from build123d import *

# Parameters (mm, degrees)
F0_R     = 25.4
F1_DEPTH = 6.35
F3_DEPTH = 12.7
F5_COUNT = 6
F6_R     = 5.616515
F7_DEPTH = 12.7


with BuildPart() as f1:
    # F0 (on Top) → F1 (new body, symmetric)
    with BuildSketch(Plane.XY):
        Circle(F0_R)
    extrude(amount=F1_DEPTH, both=True)

    # F2 (on face) → F3 (join)
    with BuildSketch(Plane(origin=(0, 0, -6.35), x_dir=(1, 0, 0), z_dir=(0, 0, -1))):
        with BuildLine():
            Line((-6.574004, 24.534516), (0, 24.477616))
            Line((0, 24.477616), (0, 25.4))
            ThreePointArc((0, 25.4), (-3.315365, 25.182699), (-6.574004, 24.534516))
        make_face()
        with BuildLine():
            Line((0, 25.4), (0, 24.477616))
            Line((0, 24.477616), (6.543582, 24.420979))
            Line((6.543582, 24.420979), (6.574004, 24.534516))
            ThreePointArc((6.574004, 24.534516), (3.315365, 25.182699), (0, 25.4))
        make_face()
        with BuildLine():
            Line((-6.486069, 34.694135), (-6.574004, 24.534516))
            ThreePointArc((-6.574004, 24.534516), (-3.315365, 25.182699), (0, 25.4))
            ThreePointArc((0, 25.4), (3.315365, 25.182699), (6.574004, 24.534516))
            Line((6.574004, 24.534516), (7.085632, 34.576668))
            Line((7.085632, 34.576668), (-6.486069, 34.694135))
        make_face()
    extrude(amount=-F3_DEPTH)

    # F5: F1 ×6 about axis
    f5_axis = Axis((0, 0, 22.241494), (0, 0, 1))


with BuildPart() as f1_1:
    add(f1.part)
    for i in range(1, F5_COUNT):
        add(f1.part.rotate(f5_axis, i * 360 / F5_COUNT))

    # F6 (on face) → F7 (cut)
    with BuildSketch(Plane.XY.offset(6.35)):
        with Locations((-0.299782, 0)):
            Circle(F6_R)
    extrude(amount=-F7_DEPTH, mode=Mode.SUBTRACT)


solid = f1_1.part
Input: part model. Units: mm. Frame: model coordinates. A direction names the side the tool comes from. Round coordinates to 2 decimals unless told otherwise and drop trailing zeros. Order: outer loops, then holes, each group sorted by start corner. A loop starts at its lowest first (then second) coordinate and runs counter-clockwise, first axis right, second up. Notation, with made-up numbers: (-12.75, -20.5) - (-1.75, -20.5) arc R11 cw to (-1.75, -4.5) - close; hole circle Ø5 at (67.5, -28). An arc over 180 degrees is marked (long way). Answer as a JSON object with one key per item and string values. Group by question number.
(1) Pin query (flat end, axial travel): P1, Ø6.5, axis at x = -0.3, y = 0, coming from the -Z side; P2, Ø1.5, axis at x = -19.5, z = 5, coming from the +Y side; P3, Ø5, axis at y = 4, z = 4.5, coming from the -X side; P4, Ø4, axis at y = -16.5, z = 5, coming from the -X side. Return the tip coordinate at first contact, or that it passes through.
(2) Cut plane A-A (y = 0). Return loops of the section in (x, z), then the cut area to 4 significant figures.
(3) Material intervals for probe 1 along X at (y, z) = (-22, 5.75); probe 2 along Y at (x, z) = (2, 2.25); probe 3 along Y at (x, z) = (28, 4.75) (3 decimals), sorted ascending. Write a range as from..to.
(4) Cut plane C-C (x = 4). Return loops of the section in (y, z), then the cut area to 3 significant figures.
(5) Draft query along Y for faces 6 (the face through (-1.03, 5.57, 0.09)), 7 (the face through (30.19, -16.98, -0.09)), 8 (the face through (22.122, 20.654, -0.089)). Return one class per face: released by +Y, released by -Y, zero draft, split by the parting line, or undercut.
(6) Cut plane D-D (x = 20). Return loops of the section in (y, z).
(7) Reachability of faces 1 (the face through (-28.95, 8.83, -0.09)), 2 (the face through (28.95, -8.83, -0.09)), 3 (the face through (29.797, 17.659, -0.089)), 4 (the face through (12.78, 21.95, 0.09)), 5 (the face through (-12.78, -21.95, 0.09)) from +Z, -Z, +X, -X, +Y, -Y: full face, straight path, thin tool, end or side. Return the list, or none.
(8) Cut plane B-B (z = 0). Return loops of the section in (x, y).
Here are the results:
{
 "1": {"P1": "passes through", "P2": "stops at y = 19.26", "P3": "stops at x = -25.36", "P4": "stops at x = -31.66"},
 "2": {"outline": "(-25.4, -6.35) - (-5.92, -6.35) - (-5.92, 6.35) - (-25.4, 6.35) - close; (5.32, -6.35) - (25.4, -6.35) - (25.4, 6.35) - (5.32, 6.35) - close", "area": "502.5 mm^2"},
 "3": {"probe 1": "x = -27.24..-24.2, -12.69..12.69, 25.1..27.35", "probe 2": "y = -34.62..-5.12, 5.12..34.66", "probe 3": "y = -20.849..-8.346, 8.615..20.71"},
 "4": {"outline": "(-34.6, -6.35) - (-3.61, -6.35) - (-3.61, 6.35) - (-34.6, 6.35) - close; (3.61, -6.35) - (34.67, -6.35) - (34.67, 6.35) - (3.61, 6.35) - close", "area": "788 mm^2"},
 "5": {"face 6": "undercut", "face 7": "released by -Y", "face 8": "released by +Y"},
 "6": {"outline": "(-19.11, -6.35) - (19.28, -6.35) - (19.28, 6.35) - (-19.11, 6.35) - close"},
 "7": {"face 1": "+Z, -Z, -X", "face 2": "+Z, -Z, +X", "face 3": "+Z, -Z, +X, +Y", "face 4": "+Z, -Z, +Y", "face 5": "+Z, -Z, -Y"},
 "8": {"outline": "(-33.49, 11.15) - (-24.53, 6.57) arc R25.4 ccw to (-24.53, -6.57) - (-33.29, -11.73) - (-26.4, -23.42) - (-17.96, -17.96) arc R25.4 ccw to (-6.57, -24.53) - (-6.49, -34.69) - (7.09, -34.58) - (6.57, -24.53) arc R25.4 ccw to (17.96, -17.96) - (26.8, -22.96) - (33.49, -11.15) - (24.53, -6.57) arc R25.4 ccw to (24.53, 6.57) - (33.29, 11.73) - (26.4, 23.42) - (17.96, 17.96) arc R25.4 ccw to (6.57, 24.53) - (6.49, 34.69) - (-7.09, 34.58) - (-6.57, 24.53) arc R25.4 ccw to (-17.96, 17.96) - (-26.8, 22.96) - close; hole circle Ø11.23 at (-0.3, 0)"}
}
